```python
from build123d import *

# Parameters (mm, degrees)
SKETCH1_W           = 62.5
SKETCH1_H           = 45
BOSS_EXTRUDE1_DEPTH = 20
CUT_EXTRUDE10_DEPTH = 59.322915736
SKETCH18_W          = 37.5
SKETCH18_H          = 20
CUT_EXTRUDE13_DEPTH = 59.322915736
SKETCH19_R          = 2.75
CUT_EXTRUDE14_DEPTH = 59.322915736
SKETCH20_R          = 1.375
CUT_EXTRUDE15_DEPTH = 80.569152314
FILLET1_R           = 2
SKETCH21_R          = 3.75
CUT_EXTRUDE16_DEPTH = 3


with BuildPart() as part:
    # Sketch1 → Boss-Extrude1 (new body)
    with BuildSketch(Plane.XY):
        with Locations((0, 22.5)):
            Rectangle(SKETCH1_W, SKETCH1_H)
    extrude(amount=BOSS_EXTRUDE1_DEPTH)

    # Sketch14 → Cut-Extrude10 (cut, through all)
    with BuildSketch(Plane.XY.offset(20)):
        with BuildLine():
            ThreePointArc((24.5, 4.288691855), (24.749252587, 4.259687402), (25, 4.25))
            Line((25, 4.25), (25, 10.75))
            ThreePointArc((25, 10.75), (21.759687402, 7.750747413), (24.5, 4.288691855))
        make_face()
        with BuildLine():
            Line((25, 10.75), (25, 4.25))
            ThreePointArc((25, 4.25), (25.250747413, 4.259687402), (25.5, 4.288691855))
            ThreePointArc((25.5, 4.288691855), (27.468552207, 5.386058184), (28.25, 7.5))
            ThreePointArc((28.25, 7.5), (27.298097039, 9.798097039), (25, 10.75))
        make_face()
        with BuildLine():
            Line((24.5, 0), (25, 0))
            Line((25, 0), (25, 4.25))
            ThreePointArc((25, 4.25), (24.749252587, 4.259687402), (24.5, 4.288691855))
            Line((24.5, 4.288691855), (24.5, 0))
        make_face()
        with BuildLine():
            Line((25, 4.25), (25, 0))
            Line((25, 0), (25.5, 0))
            Line((25.5, 0), (25.5, 4.288691855))
            ThreePointArc((25.5, 4.288691855), (25.250747413, 4.259687402), (25, 4.25))
        make_face()
    cut_extrude10 = extrude(amount=-CUT_EXTRUDE10_DEPTH, mode=Mode.SUBTRACT)

    # Mirror1: Cut-Extrude10 across plane
    add(cut_extrude10.mirror(Plane(origin=(0, 0, 0), x_dir=(0, 0, 1), z_dir=(1, 0, 0))), mode=Mode.SUBTRACT)

    # Sketch18 → Cut-Extrude13 (cut, through all)
    with BuildSketch(Plane.XY.offset(20)):
        with Locations((0, 10)):
            Rectangle(SKETCH18_W, SKETCH18_H)
    extrude(amount=-CUT_EXTRUDE13_DEPTH, mode=Mode.SUBTRACT)

    # Sketch19 → Cut-Extrude14 (cut, through all)
    with BuildSketch(Plane.XY.offset(20)):
        with Locations((0, 27.5)):
            Circle(SKETCH19_R)
    extrude(amount=-CUT_EXTRUDE14_DEPTH, mode=Mode.SUBTRACT)

    # Sketch20 → Cut-Extrude15 (cut, through all)
    with BuildSketch(Plane(origin=(31.25, 0, 0), x_dir=(0, 0, -1), z_dir=(1, 0, 0))):
        with Locations(Location((-5, 2.5, 0), (0, 0, 180))):
            Circle(SKETCH20_R)
        with Locations(Location((-15, 2.5, 0), (0, 0, 180))):
            Circle(SKETCH20_R)
    extrude(amount=-CUT_EXTRUDE15_DEPTH, mode=Mode.SUBTRACT)

    # Fillet1
    # the kernel refuses this fillet: 2 mm, written as the material it takes off along each edge
    with BuildSketch(Plane(origin=(31.25, 0, -5), x_dir=(0, 1, 0), z_dir=(0, 0, 1)), Plane(origin=(-31.25, 0, -5), x_dir=(1, 0, 0), z_dir=(0, 0, 1))) as fillet1_piece_1:
        with BuildLine():
            CenterArc((FILLET1_R, FILLET1_R), FILLET1_R, 180, 90)
            Line((0, FILLET1_R), (0, 0))
            Line((0, 0), (FILLET1_R, 0))
        make_face()
    extrude(amount=30, mode=Mode.SUBTRACT)

    # Sketch21 → Cut-Extrude16 (cut)
    with BuildSketch(Plane(origin=(31.25, 0, 0), x_dir=(0, 0, -1), z_dir=(1, 0, 0))):
        with Locations((-5, 2.5)):
            Circle(SKETCH21_R)
        with Locations((-15, 2.5)):
            Circle(SKETCH21_R)
    cut_extrude16 = extrude(amount=-CUT_EXTRUDE16_DEPTH, mode=Mode.SUBTRACT)

    # Mirror2: Cut-Extrude16 across plane
    add(cut_extrude16.mirror(Plane(origin=(0, 0, 0), x_dir=(0, 0, 1), z_dir=(1, 0, 0))), mode=Mode.SUBTRACT)


solid = part.part
```
Read the model definition and answer for the solid it produces. Units are mm, in the model's axes. A direction names the side the tool comes from. Coordinates: 2 decimals unless noted, no trailing zeros. Order: outer loops, then holes, each group sorted by start corner. A loop starts at its lowest first (then second) coordinate and runs counter-clockwise, first axis right, second up. Notation, with made-up numbers: (26.5, 54) - (78.5, 54) arc R18 ccw to (78.5, 67) - close; hole circle Ø5 at (-13.5, 50). An arc over 180 degrees is marked (long way). Answer as a JSON object with one key per item and string values. Group by question number.
Item 1: Consider probe 1 along X at (y, z) = (2, 3); probe 2 along Z at (x, y) = (-27.5, 2.5) (3 decimals); probe 3 along Y at (x, z) = (20.1, 15) (3 decimals). Determine where each line is inside the solid, lowest interval first. Write a range as from..to.
Item 2: Section D-D (z = 5) is taken. State how many separate pieces and enclosed holes the cut face has, plus the area to 3 significant figures.
Item 3: A tool of negligible diameter and unlimited length cuts with its end or side. For faces 4 (the face through (-24.5, 2, 10)), 5 (the face through (0, 23, 20)), 6 (the face through (-0.358, 30.227, 10.14)), 7 (the face through (-29.77, 6.25, 14.88)), 8 (the face through (28.25, 4, 14)), from which of +Z, -Z, +X, -X, +Y, -Y can it reach the whole face along a straight path? Write none if from no direction.
Item 4: The mould has two halves that part along X. Classify faces 1 (the face through (-30.415, 0.374, 9.969)), 2 (the face through (-22, 0, 10)), 3 (the face through (-25.5, 2, 10)): +X half, -X half, draft (parallel to the pull), parting line (faces both ways), or undercut.
Item 5: Section C-C (x = -27) is taken. Give the vertices of the cut face in (y, z) (3 decimals).
Item 6: Flat-ended cylindrical pins translate along their axes: P1, Ø4.5, axis at y = 2.5, z = 15, coming from the +X side; P2, Ø5, axis at x = 0, y = 27.5, coming from the -Z side; P3, Ø4.5, axis at y = 2.5, z = 15, coming from the -X side. Find the tip coordinate at first contact, or state that the pin passes through.
Item 7: Section A-A (x = 0) is taken. Give the vertices of the cut face in (y, z).
Item 8: Section B-B (y = 27.5) is taken. Give the vertices of the cut face in (x, z).
Results are:
{
 "1": {"probe 1": "x = -28.25..-25.5, -24.5..-18.75, 18.75..24.5, 25.5..28.25", "probe 2": "z = 0..3.625, 6.375..13.625, 16.375..20", "probe 3": "y = 0..1.125, 3.875..45"},
 "2": {"separate pieces": "5", "enclosed holes": "1", "area": "1,880 mm^2"},
 "3": {"face 4": "+Z, -Z, -Y", "face 5": "+Z, +X, -X, +Y, -Y", "face 6": "+Z, -Z", "face 7": "-X", "face 8": "+X"},
 "4": {"face 1": "-X half", "face 2": "draft", "face 3": "undercut"},
 "5": {"outline": "(0, 0) - (4.938, 0) - (4.938, 20) - (0, 20) - close; (10.062, 0) - (45, 0) - (45, 20) - (10.062, 20) - close; hole circle Ø2.75 at (2.5, 5); hole circle Ø2.75 at (2.5, 15)"},
 "6": {"P1": "stops at x = 28.25", "P2": "passes through", "P3": "stops at x = -28.25"},
 "7": {"outline": "(20, 0) - (24.75, 0) - (24.75, 20) - (20, 20) - close; (30.25, 0) - (45, 0) - (45, 20) - (30.25, 20) - close"},
 "8": {"outline": "(-31.25, 0) - (-2.75, 0) - (-2.75, 20) - (-31.25, 20) - close; (2.75, 0) - (31.25, 0) - (31.25, 20) - (2.75, 20) - close"}
}
